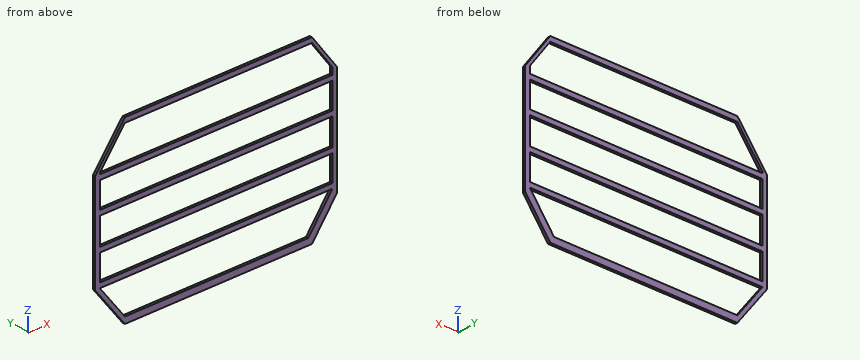
```python
from build123d import *

# Parameters (mm, degrees)
BOSS_EXTRUDE1_DEPTH = 10
CUT_EXTRUDE1_DEPTH  = 10
BOSS_EXTRUDE3_START = -20
SKETCH7_W           = 80
SKETCH7_H           = 80
BOSS_EXTRUDE3_DEPTH = 30
SKETCH8_W           = 925.61
SKETCH8_H           = 100
SKETCH8_H_2         = 104.39
SKETCH8_W_2         = 80
SKETCH8_H_3         = 80
CUT_EXTRUDE6_DEPTH  = 10


with BuildPart() as part:
    # Sketch2 → Boss-Extrude1 (new body)
    with BuildSketch(Plane(origin=(0, 0, 0), x_dir=(1, 0, 0), z_dir=(0, 1, 0))):
        Polygon((118.58, 345.487717935), (863.58, 345.487717935), (963.71, 209.828898833), (963.71, -209.828898833), (863.58, -345.487717935), (118.58, -345.487717935), (0, -190.295), (0, 190.295), align=None)
    extrude(amount=BOSS_EXTRUDE1_DEPTH)

    # Sketch3 → Cut-Extrude1 (cut)
    with BuildSketch(Plane(origin=(0, 10, 0), x_dir=(1, 0, 0), z_dir=(0, 1, 0))):
        with BuildLine():
            Line((340, -245.487717935), (340, -279.772016162))
            Line((340, -279.772016162), (341.671796469, -281.959995904))
            ThreePointArc((341.671796469, -281.959995904), (371.660256421, -306.647976918), (409.484364019, -315.487717935))
            Line((409.484364019, -315.487717935), (542.385502063, -315.487717935))
            Line((542.385502063, -315.487717935), (542.385502063, -245.487717935))
            Line((542.385502063, -245.487717935), (340, -245.487717935))
        make_face()
    cut_extrude1 = extrude(amount=-CUT_EXTRUDE1_DEPTH, mode=Mode.SUBTRACT)

    # Sketch7 → Boss-Extrude3 (add)
    with BuildSketch(Plane(origin=(0, 10, 0), x_dir=(1, 0, 0), z_dir=(0, 1, 0)).offset(BOSS_EXTRUDE3_START)):
        with Locations((89.309431631, -0.676064103)):
            Rectangle(SKETCH7_W, SKETCH7_H)
    boss_extrude3 = extrude(amount=BOSS_EXTRUDE3_DEPTH)

    # Mirror2: Boss-Extrude3 across plane
    add(boss_extrude3.mirror(Plane.ZY.offset(-481.855)))

    # Mirror3: Cut-Extrude1 across plane
    add(cut_extrude1.mirror(Plane.XY), mode=Mode.SUBTRACT)

    # Sketch8 → Cut-Extrude6 (cut)
    with BuildSketch(Plane(origin=(0, 10, 0), x_dir=(1, 0, 0), z_dir=(0, 1, 0))):
        Polygon((848.514252318, 320.555846821), (118.58, 320.555846821), (19.05, 190.295), (944.66, 190.295), align=None)
        with BuildLine():
            Line((409.484364019, 315.487717935), (542.385502063, 315.487717935))
            Line((542.385502063, 315.487717935), (542.385502063, 245.487717935))
            Line((542.385502063, 245.487717935), (340, 245.487717935))
            Line((340, 245.487717935), (340, 279.772016162))
            Line((340, 279.772016162), (341.671796469, 281.959995904))
            ThreePointArc((341.671796469, 281.959995904), (371.660256421, 306.647976918), (409.484364019, 315.487717935))
        make_face(mode=Mode.SUBTRACT)
        with Locations((481.855, 121.245)):
            Rectangle(SKETCH8_W, SKETCH8_H)
        with Locations((481.855, 0)):
            Rectangle(SKETCH8_W, SKETCH8_H_2)
        with Locations((89.309431631, -0.676064103)):
            Rectangle(SKETCH8_W_2, SKETCH8_H_3, mode=Mode.SUBTRACT)
        with Locations((874.400568369, -0.676064103)):
            Rectangle(SKETCH8_W_2, SKETCH8_H_3, mode=Mode.SUBTRACT)
        with Locations((481.855, -121.245)):
            Rectangle(SKETCH8_W, SKETCH8_H)
        Polygon((944.66, -190.295), (19.05, -190.295), (19.05, -196.176871114), (118.58, -326.437717935), (863.58, -326.437717935), (944.66, -216.588351584), align=None)
        with BuildLine():
            Line((340, -279.772016162), (340, -245.487717935))
            Line((340, -245.487717935), (542.385502063, -245.487717935))
            Line((542.385502063, -245.487717935), (542.385502063, -315.487717935))
            Line((542.385502063, -315.487717935), (409.484364019, -315.487717935))
            ThreePointArc((409.484364019, -315.487717935), (371.660256421, -306.647976918), (341.671796469, -281.959995904))
            Line((341.671796469, -281.959995904), (340, -279.772016162))
        make_face(mode=Mode.SUBTRACT)
    extrude(amount=-CUT_EXTRUDE6_DEPTH, mode=Mode.SUBTRACT)


with BuildPart() as body_2:
    # of the pieces the cut leaves, the one that is kept (cut_extrude6_keep)
    add(part.part.solids().sort_by_distance((118.58, 0, -345.487717935))[0])


solid = body_2.part
```
Work out the finished part from the listing and answer in its coordinate system (mm). Round coordinates to 2 decimals unless told otherwise and drop trailing zeros. Write each loop counter-clockwise with the first axis right and the second up, starting at its lowest first coordinate (ties: lowest second). Pieces come first, ordered by that corner, then holes. Notation, with made-up numbers: (25, 45.25) - (60, 45.25) arc R21 cw to (60, 73.25) - close; hole circle Ø1 at (59.5, 77). An arc over 180 degrees is marked (long way). Return JSON: item names as keys, results as strings. Group by question number.
Q1. The part is cut by section A-A on x = 817.5. Write down the section's boundary in (y, z) (3 decimals).
Q2. Find the intervals of material crossed by L1, parallel to Z at x = 572.5, y = 5.75 (3 decimals); L2, parallel to X at y = 7.25, z = 2.5; L3, parallel to Z at x = 109, y = 6.25 (3 decimals), in increasing order.
Q3. Each of these flat-tipped pins is pushed along its axis until it touches: pin 1 Ø3 at (y, z) = (7.5, -119.5) entering from -X; pin 2 Ø5 at (y, z) = (3, 201.5) entering from -X. Where does it stop, or does it pass through?
Q4. The part is cut by section D-D on z = -278.5. Write down the section's boundary in (x, y).
Q5. The part is cut by section B-B on y = 2.25. Count the separate pieces of the cut face and the enclosed holes in it, then the cut area to 3 significant figures.
Q6. The part is cut by section C-C on z = 139. Write down the section's boundary in (x, y).
Solved:
{
 "1": {"outline": "(0, -345.488) - (10, -345.488) - (10, -320.556) - (0, -320.556) - close; (0, -190.295) - (10, -190.295) - (10, -171.245) - (0, -171.245) - close; (0, -71.245) - (10, -71.245) - (10, -52.195) - (0, -52.195) - close; (0, 52.195) - (10, 52.195) - (10, 71.245) - (0, 71.245) - close; (0, 171.245) - (10, 171.245) - (10, 190.295) - (0, 190.295) - close; (0, 326.438) - (10, 326.438) - (10, 345.488) - (0, 345.488) - close"},
 "2": {"L1": "-345.488 to -320.556, -190.295 to -171.245, -71.245 to -52.195, 52.195 to 71.245, 171.245 to 190.295, 326.438 to 345.488", "L2": "0 to 19.05, 944.66 to 963.71", "L3": "-332.95 to -308.018, -190.295 to -171.245, -71.245 to -52.195, 52.195 to 71.245, 171.245 to 190.295, 313.9 to 332.95"},
 "3": {"pin 1": "x = 0", "pin 2": "x = 6.65"},
 "4": {"outline": "(67.4, 0) - (86.45, 0) - (86.45, 10) - (67.4, 10) - close; (879.56, 0) - (913.02, 0) - (913.02, 10) - (879.56, 10) - close"},
 "5": {"separate pieces": "1", "enclosed holes": "5", "area": "129,000 mm²"},
 "6": {"outline": "(0, 0) - (19.05, 0) - (19.05, 10) - (0, 10) - close; (944.66, 0) - (963.71, 0) - (963.71, 10) - (944.66, 10) - close"}
}
